```python
from build123d import *

# Parameters (mm, degrees)
SKETCH1_W                = 71.755
SKETCH1_H                = 50.8
MAIN_BODY_DEPTH          = 3.175
SKETCH2_W                = 3.2258
SKETCH2_H                = 6.35
SKETCH2_W_2              = 6.35
SKETCH2_H_2              = 3.2258
TABS_DEPTH               = 3.175
NOSE_SECTION_DEPTH       = 3.175
SKETCH8_R                = 0.508
CUT_FOR_MOTORS_DEPTH     = 4.1750001
SLOT_FOR_FIREWALL_DEPTH  = 4.1750001
EXTENSION_FOR_AXLE_DEPTH = 3.175
SKETCH11_R               = 3.2385
CUT_FOR_AXLE_DEPTH       = 4.1750001


with BuildPart() as part:
    # Sketch1 → main body (new body)
    with BuildSketch(Plane(origin=(0, 0, 0), x_dir=(0, 0, -1), z_dir=(1, 0, 0))):
        Rectangle(SKETCH1_W, SKETCH1_H)
    extrude(amount=MAIN_BODY_DEPTH)

    # Sketch2 → tabs (add)
    with BuildSketch(Plane(origin=(3.175, 0, 0), x_dir=(0, 0, -1), z_dir=(1, 0, 0))):
        with Locations((-37.4904, 16.256)):
            Rectangle(SKETCH2_W, SKETCH2_H)
        with Locations((37.4904, 15.875)):
            Rectangle(SKETCH2_W, SKETCH2_H)
        with Locations((37.4904, -15.875)):
            Rectangle(SKETCH2_W, SKETCH2_H)
        with Locations((14.9225, -27.0129)):
            Rectangle(SKETCH2_W_2, SKETCH2_H_2)
    extrude(amount=-TABS_DEPTH)

    # Sketch3 → nose section (add)
    with BuildSketch(Plane.ZY):
        with BuildLine():
            Line((51.326941337, -21.081213956), (45.4025, -21.081213956))
            Line((45.4025, -21.081213956), (45.4025, 4.459215194))
            Line((45.4025, 4.459215194), (39.534554548, 6.35))
            Line((39.534554548, 6.35), (35.8775, 6.35))
            Line((35.8775, 6.35), (35.8775, -25.4))
            Line((35.8775, -25.4), (35.8775, -57.323174337))
            Line((35.8775, -57.323174337), (42.8625, -65.53778801))
            Line((42.8625, -65.53778801), (51.326941337, -65.53778801))
            Line((51.326941337, -65.53778801), (71.872461292, -61.17070293))
            add(Edge.make_bspline(
                [(71.573902629, -54.710271069), (74.102249919, -57.868358167), (71.872461292, -61.17070293)],
                knots=[0, 0, 0, 1, 1, 1], degree=2))
            add(Edge.make_bspline(
                [(71.573902629, -54.710271069), (65.707060229, -46.091929926), (62.410515677, -39.350220463), (53.353361757, -23.389519751), (51.326941337, -21.081213956)],
                knots=[0, 0, 0, 0, 0.673726306, 1, 1, 1, 1], degree=3))
        make_face()
    extrude(amount=-NOSE_SECTION_DEPTH)

    # Sketch8 → cut for motors (cut, through all)
    with BuildSketch(Plane.ZY):
        with Locations((-26.9875, 0.508)):
            Circle(SKETCH8_R)
        with Locations((0.9525, 0.508)):
            Circle(SKETCH8_R)
        with Locations((-26.9875, -16.002)):
            Circle(SKETCH8_R)
        with Locations((0.9525, -16.002)):
            Circle(SKETCH8_R)
        Polygon((-1.5875, -5.842), (-1.5875, 6.858), (-24.4475, 6.858), (-24.4475, 3.683), (-25.8445, 3.683), (-25.8445, -2.667), (-24.4475, -2.667), (-24.4475, -5.842), align=None)
        Polygon((-1.5875, -22.352), (-1.5875, -9.652), (-24.4475, -9.652), (-24.4475, -12.827), (-25.8445, -12.827), (-25.8445, -19.177), (-24.4475, -19.177), (-24.4475, -22.352), align=None)
    extrude(amount=-CUT_FOR_MOTORS_DEPTH, mode=Mode.SUBTRACT)

    # Sketch9 → slot for firewall (cut, through all)
    with BuildSketch(Plane.ZY):
        Polygon((20.5105, -6.34593574), (23.6855, -6.34593574), (23.6855, 12.7), (32.7025, 25.4), (23.1775, 25.4), (20.0025, 25.4), (10.4775, 25.4), (20.5105, 12.70406426), align=None)
    extrude(amount=-SLOT_FOR_FIREWALL_DEPTH, mode=Mode.SUBTRACT)

    # Sketch10 → extension for axle (add)
    with BuildSketch(Plane.ZY):
        Polygon((35.8775, -57.323174337), (35.8775, -25.4), (8.5725, -25.4), (8.5725, -65.53778801), (42.8625, -65.53778801), align=None)
    extrude(amount=-EXTENSION_FOR_AXLE_DEPTH)

    # Sketch11 → cut for axle (cut, through all)
    with BuildSketch(Plane.ZY):
        with Locations((18.2245, -55.753)):
            Circle(SKETCH11_R)
    extrude(amount=-CUT_FOR_AXLE_DEPTH, mode=Mode.SUBTRACT)


solid = part.part
```
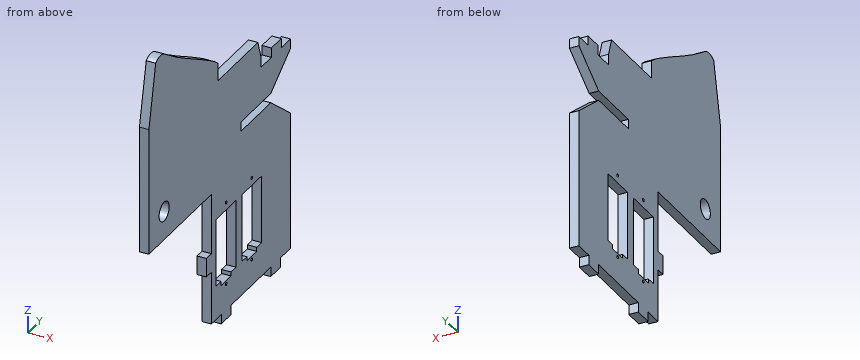
CAD build for the part. Positions are in the model's coordinates, mm. Coordinates: 2 decimals unless noted, no trailing zeros. Order: outer loops, then holes, each group sorted by start corner. A loop starts at its lowest first (then second) coordinate and runs counter-clockwise, first axis right, second up. Notation, with made-up numbers: (-20.5, -28) -> (26.5, -28) arc R33 cw to (26.5, 9) -> close; hole circle Ø1 at (71.5, 68.25). An arc over 180 degrees is marked (long way). Use one line per item in the form item = value. Start each with the question number.
1) Drop flat-ended pins along their axis: pin 1 (1 mm diameter, centred on x = 1, y = 23, fed in from -Z); pin 2 (1 mm diameter, centred on x = 1.5, z = -10, fed in from -Y); pin 3 (6 mm diameter, centred on y = -55.75, z = 18.22, fed in from -X); pin 4 (1.6 mm diameter, centred on x = 1.5, y = -8.5, fed in from +Z). Give the stop position or say it passes through.
2) Band-saw the part on B-B on y = -8. Give the cut face in (x, z) (1 decimal).
3) Band-saw the part on A-A on z = -7. Give the cut face in (x, y) (3 decimals), then the cut area to 3 significant figures.
4) Band-saw the part on D-D on z = 31. Give the cut face in (x, y) (3 decimals).
5) Drill centre lines: L1, parallel to Y at x = 0.95, z = -15; L2, parallel to Y at x = 0.5, z = -10; L3, parallel to Y at x = 0.8, z = 39.5. Where is each one in solid material? Low to high. Write a range as [from, to].
6) Band-saw the part on C-C on x = 1.8. State how many separate pieces and enclosed holes the cut face has, then the cut area to 3 significant figures.
Entries:
q1.pin_1 = -35.88
q1.pin_2 = -25.4
q1.pin_3 = through
q1.pin_4 = 45.4
q2.outline = (0, -35.9) -> (3.2, -35.9) -> (3.2, 45.4) -> (0, 45.4) -> close
q3.outline = (0, -25.4) -> (3.175, -25.4) -> (3.175, -22.352) -> (0, -22.352) -> close; (0, -9.652) -> (3.175, -9.652) -> (3.175, -5.842) -> (0, -5.842) -> close; (0, 6.858) -> (3.175, 6.858) -> (3.175, 25.4) -> (0, 25.4) -> close
q3.area = 80.6 mm2
q4.outline = (0, -65.538) -> (3.175, -65.538) -> (3.175, 23.002) -> (0, 23.002) -> close
q5.L1 = [-28.63, -22.35], [-9.65, -5.84], [6.86, 25.4]
q5.L2 = [-25.4, -22.35], [-9.65, -5.84], [6.86, 25.4]
q5.L3 = [-65.54, 6.35]
q6.separate_pieces = 1
q6.enclosed_holes = 7
q6.area = 5,430 mm2
